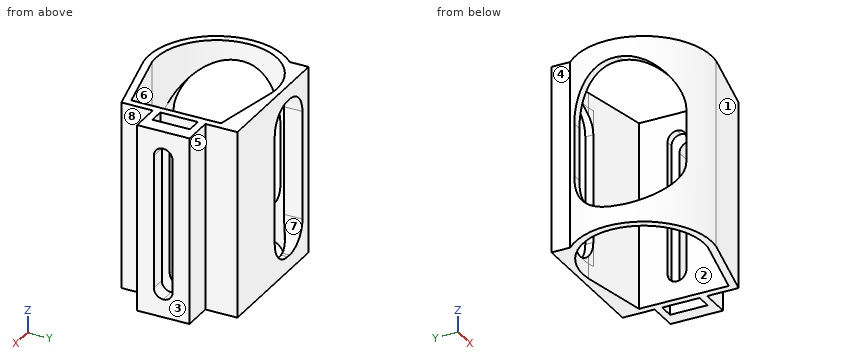
from build123d import *
from OCP.BRepAlgoAPI import BRepAlgoAPI_Cut
from OCP.TopTools import TopTools_ListOfShape

# Parameters (mm, degrees)
SALIENTE_EXTRUIR1_DEPTH     = 50
SALIENTE_EXTRUIR2_DEPTH     = 50
CORTAR_EXTRUIR12_REACH      = 77.399
REDONDEO1_R                 = 2.5
CORTAR_EXTRUIR17_REACH      = 77.931
CORTAR_EXTRUIR17_END_RADIUS = 16.15
CORTAR_EXTRUIR19_REACH      = 79.662
CROQUIS18_W                 = 7
CROQUIS18_H                 = 42
CORTAR_EXTRUIR22_REACH      = 79.662
CORTAR_EXTRUIR22_END_RADIUS = 16.15
CROQUIS22_W                 = 7
CROQUIS22_H                 = 42
REDONDEO10_START            = 3.308867588
REDONDEO10_DEPTH            = 4.936164621
REDONDEO10_START_2          = 6.105712769
REDONDEO10_2_DEPTH          = 2.13931944
REDONDEO10_START_3          = 4
REDONDEO10_3_DEPTH          = 42


with BuildPart() as part:
    # Croquis3 → Saliente-Extruir1 (new body)
    with BuildSketch(Plane.XY):
        with BuildLine():
            Line((-42.099195701, 8.245032209), (-6.157247249, 8.245032209))
            Line((-6.157247249, 8.245032209), (-6.157247249, -22.679560551))
            Line((-6.157247249, -22.679560551), (-26.590955846, -27.481197975))
            ThreePointArc((-26.590955846, -27.481197975), (-45.398833914, -17.697170572), (-42.099195701, 3.245032209))
            Line((-42.099195701, 3.245032209), (-42.099195701, 8.245032209))
        make_face()
        with BuildLine():
            Line((-8.157247249, 2.82108494), (-26.731262437, 6.441781026))
            ThreePointArc((-26.731262437, 6.441781026), (-45.345288804, -9.402744466), (-26.961453667, -25.513783269))
            Line((-26.961453667, -25.513783269), (-8.157247249, -21.095056202))
            Line((-8.157247249, -21.095056202), (-8.157247249, 2.82108494))
        make_face(mode=Mode.SUBTRACT)
    extrude(amount=SALIENTE_EXTRUIR1_DEPTH)

    # Croquis11 → Saliente-Extruir2 (add)
    with BuildSketch(Plane(origin=(0, 0, 0), x_dir=(-1, 0, 0), z_dir=(0, 0, -1))):
        Polygon((-1.842752751, -14.302804028), (-1.842752751, -0.302804028), (6.157247249, -0.302804028), (6.157247249, -2.302804028), (2.157247249, -2.302804028), (2.157247249, -12.302804028), (6.157247249, -12.302804028), (6.157247249, -14.302804028), align=None)
    extrude(amount=-SALIENTE_EXTRUIR2_DEPTH)

    # Cortar-Extruir12: up to this face of the body (flat: up to its plane)
    cortar_extruir12_end = Plane(part.part.faces().sort_by_distance((-8.157247249, -9.136985631, 25))[0])
    # Croquis12 → Cortar-Extruir12 (cut, up to the picked face)
    with BuildSketch(Plane(origin=(1.842752751, 0, 0), x_dir=(0, 0, -1), z_dir=(1, 0, 0)), mode=Mode.PRIVATE) as cortar_extruir12_sk1:
        Polygon((-25, -9.802804028), (-4.8, -9.802804028), (-4.8, -4.802804028), (-45.42287301, -4.802804028), (-45.42287301, -9.802804028), align=None)
    cortar_extruir12_tool1 = split(extrude(cortar_extruir12_sk1.sketch, amount=-CORTAR_EXTRUIR12_REACH, mode=Mode.PRIVATE), bisect_by=cortar_extruir12_end, keep=Keep.BOTH, mode=Mode.PRIVATE)
    add(cortar_extruir12_tool1.solids().sort_by(Axis((1.842753, -7.302804, 25.111437), (-1, 0, 0)))[0], mode=Mode.SUBTRACT)

    # Redondeo1
    redondeo1_edges = [part.edges().sort_by_distance(p)[0] for p in [
        (-0.157247249, -4.802804028, 4.8),
        (-0.157247249, -9.802804028, 4.8),
        (-0.157247249, -9.802804028, 45.42287301),
        (-0.157247249, -4.802804028, 45.42287301),
        (-7.157247249, -9.802804028, 4.8),
        (-7.157247249, -4.802804028, 4.8),
        (-7.157247249, -9.802804028, 45.42287301),
        (-7.157247249, -4.802804028, 45.42287301),
    ]]
    fillet(redondeo1_edges, radius=REDONDEO1_R - 0.0001)  # a hair under: the kernel refuses the full size

    # Cortar-Extruir17: up to this cylinder (the profile starts outside it)
    cortar_extruir17_end = Plane(origin=(-29.1957078, -9.519077631, 25), z_dir=(0, 0, -1)) * Cylinder(CORTAR_EXTRUIR17_END_RADIUS, 189.162, mode=Mode.PRIVATE)
    # Croquis16 → Cortar-Extruir17 (cut, up to the surface)
    with BuildSketch(Plane.ZY.offset(48.157247249), mode=Mode.PRIVATE) as cortar_extruir17_sk1:
        with BuildLine():
            Line((32, -25.481197975), (18, -25.481197975))
            ThreePointArc((18, -25.481197975), (8.807611845, -21.67358613), (5, -12.481197975))
            Line((5, -12.481197975), (5, -11.754967791))
            ThreePointArc((5, -11.754967791), (8.807611845, -2.562579636), (18, 1.245032209))
            Line((18, 1.245032209), (32, 1.245032209))
            ThreePointArc((32, 1.245032209), (41.192388155, -2.562579636), (45, -11.754967791))
            Line((45, -11.754967791), (45, -12.481197975))
            ThreePointArc((45, -12.481197975), (41.192388155, -21.67358613), (32, -25.481197975))
        make_face()
    cortar_extruir17_tool1 = extrude(cortar_extruir17_sk1.sketch, amount=-CORTAR_EXTRUIR17_REACH, mode=Mode.PRIVATE) - cortar_extruir17_end
    add(cortar_extruir17_tool1.solids().sort_by_distance((-48.157247, -12.118083, 25))[0], mode=Mode.SUBTRACT)

    # Croquis18 → Cortar-Extruir19 (cut, up to next)
    with BuildSketch(Plane(origin=(0, 8.245032209, 0), x_dir=(1, 0, 0), z_dir=(0, 1, 0)), mode=Mode.PRIVATE) as cortar_extruir19_sk1:
        with Locations((-28.507247249, -25)):
            Rectangle(CROQUIS18_W, CROQUIS18_H)
    cortar_extruir19_tool1 = extrude(cortar_extruir19_sk1.sketch, amount=-CORTAR_EXTRUIR19_REACH, mode=Mode.PRIVATE) & part.part
    add(cortar_extruir19_tool1.solids().sort_by_distance((-28.507247, 8.245032, 25))[0], mode=Mode.SUBTRACT)

    # Cortar-Extruir22: up to this cylinder (the profile starts outside it)
    cortar_extruir22_end = Plane(origin=(-29.1957078, -9.519077631, 25), z_dir=(0, 0, -1)) * Cylinder(CORTAR_EXTRUIR22_END_RADIUS, 192.624, mode=Mode.PRIVATE)
    # Croquis22 → Cortar-Extruir22 (cut, up to the surface)
    with BuildSketch(Plane(origin=(0, 8.245032209, 0), x_dir=(1, 0, 0), z_dir=(0, 1, 0)), mode=Mode.PRIVATE) as cortar_extruir22_sk1:
        with Locations((-35.507247249, -25)):
            Rectangle(CROQUIS22_W, CROQUIS22_H)
    cortar_extruir22_tool1 = extrude(cortar_extruir22_sk1.sketch, amount=-CORTAR_EXTRUIR22_REACH, mode=Mode.PRIVATE) - cortar_extruir22_end
    add(cortar_extruir22_tool1.solids().sort_by_distance((-35.507247, 8.245032, 25))[0], mode=Mode.SUBTRACT)


with BuildPart() as redondeo10_tool:
    # Redondeo10: read off the stored shape, not the designer's step
    # Redondeo10 outline → Redondeo10 (new body)
    with BuildSketch(Plane(origin=(0, 0, 0), x_dir=(1, 0, 0), z_dir=(0, 1, 0)).offset(REDONDEO10_START)):
        with BuildLine():
            Line((-39.007247249, -4), (-39.007247249, -10.5))
            ThreePointArc((-39.007247249, -10.5), (-37.103441327, -5.903805922), (-32.507247249, -4))
            Line((-32.507247249, -4), (-39.007247249, -4))
        make_face()
        with BuildLine():
            ThreePointArc((-32.507247249, -46), (-37.103441327, -44.096194078), (-39.007247249, -39.5))
            Line((-39.007247249, -39.5), (-39.007247249, -46))
            Line((-39.007247249, -46), (-32.507247249, -46))
        make_face()
    extrude(amount=REDONDEO10_DEPTH)


with BuildPart() as part_1:
    add(part.part)


with BuildPart() as part_2:
    # Redondeo10: joined with redondeo10_tool
    add(part_1.part.fuse(redondeo10_tool.part, tol=0.00001))


with BuildPart() as redondeo10_2_tool:
    # Redondeo10 2 outline → Redondeo10 2 (new body)
    with BuildSketch(Plane(origin=(0, 0, 0), x_dir=(1, 0, 0), z_dir=(0, 1, 0)).offset(REDONDEO10_START_2)):
        with BuildLine():
            Line((-25.007247249, -4), (-31.507247249, -4))
            ThreePointArc((-31.507247249, -4), (-26.911053171, -5.903805922), (-25.007247249, -10.5))
            Line((-25.007247249, -10.5), (-25.007247249, -4))
        make_face()
        with BuildLine():
            ThreePointArc((-25.007247249, -39.5), (-26.911053171, -44.096194078), (-31.507247249, -46))
            Line((-31.507247249, -46), (-25.007247249, -46))
            Line((-25.007247249, -46), (-25.007247249, -39.5))
        make_face()
    extrude(amount=REDONDEO10_2_DEPTH)


with BuildPart() as part_3:
    add(part_2.part)


with BuildPart() as part_4:
    # Redondeo10 2: joined with redondeo10_2_tool
    add(part_3.part.fuse(redondeo10_2_tool.part, tol=0.00001))


with BuildPart() as redondeo10_3_tool:
    # Redondeo10 3 outline → Redondeo10 3 (new body)
    with BuildSketch(Plane.XY.offset(REDONDEO10_START_3)):
        with BuildLine():
            Line((-39.007247249, 3.308868177), (-32.507247249, 3.308867588))
            Line((-32.507247249, 3.308867588), (-32.507247249, 6.287762866))
            ThreePointArc((-32.507247249, 6.287762866), (-35.924173697, 5.162551934), (-39.007247249, 3.308868177))
        make_face()
        with BuildLine():
            Line((-31.507247249, 6.105712769), (-25.007247249, 6.105712769))
            Line((-25.007247249, 6.105712769), (-26.731262437, 6.441781026))
            ThreePointArc((-26.731262437, 6.441781026), (-29.118405097, 6.630737362), (-31.507247249, 6.464641754))
            Line((-31.507247249, 6.464641754), (-31.507247249, 6.105712769))
        make_face()
    extrude(amount=REDONDEO10_3_DEPTH)


with BuildPart() as part_5:
    add(part_4.part)

    # Redondeo10 3: cut by redondeo10_3_tool, with a tolerance
    redondeo10_3_stock = TopTools_ListOfShape()
    redondeo10_3_stock.Append(part_5.part.wrapped)
    redondeo10_3_tools = TopTools_ListOfShape()
    redondeo10_3_tools.Append(redondeo10_3_tool.part.wrapped)
    redondeo10_3_cut = BRepAlgoAPI_Cut()
    redondeo10_3_cut.SetArguments(redondeo10_3_stock)
    redondeo10_3_cut.SetTools(redondeo10_3_tools)
    redondeo10_3_cut.SetFuzzyValue(0.00001)
    redondeo10_3_cut.Build()
    add(Compound.cast(redondeo10_3_cut.Shape()).solids(), mode=Mode.REPLACE)


solid = part_5.part
Design review of the part built by this model. Coordinates are the model's own, in mm. Face numbers are marked on the shaded views. A direction names the side the tool comes from. Give positions to 0.01 mm unless a question says otherwise; leave off trailing zeros. Order: outer loops, then holes, each group sorted by start corner. A loop starts at its lowest first (then second) coordinate and runs counter-clockwise, first axis right, second up. Notation, with made-up numbers: (-34.5, -1) - (-10.5, -1) arc R16 cw to (-10.5, 11) - close; hole circle Ø7 at (-13.5, -1.75). An arc over 180 degrees is marked (long way). Write item = value, one per line. Start each with the question number.
Q1. We need section A-A on x = -4.5. State the section outline as (y, z) points, plus the area to 3 significant figures.
Q2. We need section D-D on x = -28. State the section outline as (y, z) points.
Q3. To check wall thickness, follow L1, parallel to X at y = -15, z = 34; L2, parallel to Y at x = -22, z = 25; L3, parallel to Z at x = -37, y = 7.5. State the ranges of each line that lie inside material, in increasing order. Write a range as from..to.
Q4. Mouldability with a two-part tool opening along Y and no side actions: class the marked faces 1, 2 and 3 as released by +Y, released by -Y, zero draft, split by the parting line, or undercut.
Q5. Clearance check with flat-ended pins moving along their axes: pin 1 Ø3 at (y, z) = (-17.5, 39.5) entering from +X; pin 2 Ø10 at (x, z) = (-11, 44) entering from -Y; pin 3 Ø3 at (x, z) = (-30, 27) entering from +Y. State where each tip first meets the part, or that it passes through.
Q6. We need section B-B on z = 35.5. State how many separate pieces and enclosed holes the cut face has, plus the area to 3 significant figures.
Q7. Tool access review of the marked faces 4, 5, 6, 7 and 8: name each direction out of +Z, -Z, +X, -X, +Y, -Y from which nothing blocks a thin tool from reaching the whole face with its end or side.
Q8. We need section C-C on y = -1. State the section outline as (x, z) points, plus the area to 3 significant figures.
Working result:
q1.outline = (-14.3, 0) - (-12.3, 0) - (-12.3, 50) - (-14.3, 50) - close; (-2.3, 0) - (-0.3, 0) - (-0.3, 50) - (-2.3, 50) - close
q1.area = 200 mm²
q2.outline = (-27.63, 0) - (-25.62, 0) - (-25.62, 50) - (-27.63, 50) - close; (6.59, 0) - (8.25, 0) - (8.25, 5.03) - (6.59, 5.03) - close; (6.59, 44.97) - (8.25, 44.97) - (8.25, 50) - (6.59, 50) - close
q3.L1 = -8.16..-6.16
q3.L2 = -26.4..-24.35, 5.52..8.25
q3.L3 = 0..5.8, 44.2..50
q4.face_1 = released by -Y
q4.face_2 = undercut
q4.face_3 = zero draft
q5.pin_1 = -6.16
q5.pin_2 = -24.99
q5.pin_3 = -25.5
q6.separate_pieces = 3
q6.enclosed_holes = 0
q6.area = 248 mm²
q7.face_4 = +Z, -Z, -X, +Y
q7.face_5 = +Z, -Z, +X, +Y
q7.face_6 = +Z, -Z
q7.face_7 = +Y
q7.face_8 = +Z, -Z, +X, -Y
q8.outline = (-45.22, 0) - (-42.92, 0) - (-42.92, 10.7) - (-45.22, 10.7) - close; (-45.22, 39.3) - (-42.92, 39.3) - (-42.92, 50) - (-45.22, 50) - close; (-8.16, 0) - (1.84, 0) - (1.84, 50) - (-8.16, 50) - close
q8.area = 549 mm²
